from build123d import *

# Parameters (mm, degrees)
SKETCH2_W                     = 60
SKETCH2_H                     = 60
BOSS_EXTRUDE1_DEPTH           = 5
SKETCH5_W                     = 9
SKETCH5_H                     = 36
BOSS_EXTRUDE2_DEPTH           = 30
BOSS_EXTRUDE3_DEPTH           = 5
BOSS_EXTRUDE4_DEPTH           = 5
FILLET6_R                     = 7
SKETCH4_W                     = 2.25
SKETCH4_H                     = 5
M4_CLEARANCE_HOLE2_AT_2_COUNT = 2
M4_CLEARANCE_HOLE2_AT_2_PITCH = 70.710678119
M4_CLEARANCE_HOLE2_AT_3_COUNT = 2
M4_CLEARANCE_HOLE2_AT_3_PITCH = 50
M4_CLEARANCE_HOLE2_AT_4_COUNT = 2
M4_CLEARANCE_HOLE2_AT_4_PITCH = 50
SKETCH17_R                    = 4.5
CUT_EXTRUDE7_DEPTH            = 5
CUT_EXTRUDE8_DEPTH            = 3
RIB9_REACH                    = 57
SKETCH19_WALLS_W              = 3
SKETCH19_WALLS_H              = 168.00000011
FILLET7_R                     = 5
CUT_EXTRUDE10_DEPTH           = 1.5
FILLET8_R                     = 1
SKETCH23_R                    = 1.25
CUT_EXTRUDE12_DEPTH           = 76.663729878
CIRPATTERN2_COUNT             = 3
FILLET10_R                    = 2
SKETCH24_R                    = 8.875
CUT_EXTRUDE13_DEPTH           = 7
CUT_EXTRUDE14_DEPTH           = 7
FILLET11_R                    = 7
SKETCH27_W                    = 5
SKETCH27_H                    = 6.169574238
CUT_EXTRUDE17_DEPTH           = 7
CUT_EXTRUDE18_DEPTH           = 1.5
CUT_EXTRUDE19_DEPTH           = 1.5
FILLET13_R                    = 3


with BuildPart() as part:
    # Sketch2 → Boss-Extrude1 (new body)
    with BuildSketch(Plane(origin=(0, 0, 0), x_dir=(1, 0, 0), z_dir=(0, 1, 0))):
        Rectangle(SKETCH2_W, SKETCH2_H)
    extrude(amount=BOSS_EXTRUDE1_DEPTH)

    # Sketch5 → Boss-Extrude2 (add)
    with BuildSketch(Plane(origin=(0, 5, 0), x_dir=(1, 0, 0), z_dir=(0, 1, 0))):
        with Locations((-25.5, 0)):
            Rectangle(SKETCH5_W, SKETCH5_H)
    extrude(amount=BOSS_EXTRUDE2_DEPTH)

    # Sketch6 → Boss-Extrude3 (add)
    with BuildSketch(Plane.XY.offset(18)):
        Polygon((-21, 35), (30, 5), (-21, 5), align=None)
    extrude(amount=-BOSS_EXTRUDE3_DEPTH)

    # Sketch15 → Boss-Extrude4 (add)
    with BuildSketch(Plane(origin=(0, 0, -18), x_dir=(-1, 0, 0), z_dir=(0, 0, -1))):
        Polygon((21, 5), (21, 35), (-30, 5), align=None)
    extrude(amount=-BOSS_EXTRUDE4_DEPTH)

    # Fillet6
    fillet6_edges = [part.edges().sort_by_distance(p)[0] for p in [
        (0, 5, 18),
        (0, 5, -18),
    ]]
    fillet(fillet6_edges, radius=FILLET6_R)

    # Sketch4 → M4 Clearance Hole2 (revolve, cut)
    with BuildSketch(Plane(origin=(25, 5, -25), x_dir=(0, 0, 1), z_dir=(1, 0, 0))):
        with Locations((1.125, 2.5)):
            Rectangle(SKETCH4_W, SKETCH4_H)
    m4_clearance_hole2 = revolve(axis=Axis((25, 11.35, -25), (0, -1, 0)), mode=Mode.SUBTRACT)

    # M4 Clearance Hole2 at 2: M4 Clearance Hole2 ×2
    with Locations(*[Vector(-0.7071067811865476, 0, 0.7071067811865476) * (i * M4_CLEARANCE_HOLE2_AT_2_PITCH) for i in range(1, M4_CLEARANCE_HOLE2_AT_2_COUNT)]):
        add(m4_clearance_hole2, mode=Mode.SUBTRACT)

    # M4 Clearance Hole2 at 3: M4 Clearance Hole2 ×2
    with Locations(*[(-i * M4_CLEARANCE_HOLE2_AT_3_PITCH, 0, 0) for i in range(1, M4_CLEARANCE_HOLE2_AT_3_COUNT)]):
        add(m4_clearance_hole2, mode=Mode.SUBTRACT)

    # M4 Clearance Hole2 at 4: M4 Clearance Hole2 ×2
    with Locations(*[(0, 0, i * M4_CLEARANCE_HOLE2_AT_4_PITCH) for i in range(1, M4_CLEARANCE_HOLE2_AT_4_COUNT)]):
        add(m4_clearance_hole2, mode=Mode.SUBTRACT)

    # Sketch17 → Cut-Extrude7 (cut)
    with BuildSketch(Plane(origin=(0, 5, 0), x_dir=(1, 0, 0), z_dir=(0, 1, 0))):
        with Locations((25, -25)):
            Circle(SKETCH17_R)
        with Locations((-25, -25)):
            Circle(SKETCH17_R)
        with Locations((-25, 25)):
            Circle(SKETCH17_R)
        with Locations((25, 25)):
            Circle(SKETCH17_R)
    extrude(amount=CUT_EXTRUDE7_DEPTH, mode=Mode.SUBTRACT)

    # Sketch18 → Cut-Extrude8 (cut)
    with BuildSketch(Plane.XZ):
        with BuildLine():
            Line((-28, 21.989601355), (-28, -21.989601355))
            ThreePointArc((-28, -21.989601355), (-21.99479618, -21.99479618), (-21.989601355, -28))
            Line((-21.989601355, -28), (21.989601355, -28))
            ThreePointArc((21.989601355, -28), (21.99479618, -21.99479618), (28, -21.989601355))
            Line((28, -21.989601355), (28, 21.989601355))
            ThreePointArc((28, 21.989601355), (21.99479618, 21.99479618), (21.989601355, 28))
            Line((21.989601355, 28), (-21.989601355, 28))
            ThreePointArc((-21.989601355, 28), (-21.99479618, 21.99479618), (-28, 21.989601355))
        make_face()
    extrude(amount=-CUT_EXTRUDE8_DEPTH, mode=Mode.SUBTRACT)

    # Sketch19 walls → Rib9 (add, up to next)
    with BuildSketch(Plane.XZ, mode=Mode.PRIVATE) as rib9_sk1:
        with Locations((15.5, 0)):
            Rectangle(SKETCH19_WALLS_W, SKETCH19_WALLS_H)
    rib9_tool1 = extrude(rib9_sk1.sketch, amount=-RIB9_REACH, mode=Mode.PRIVATE) - part.part
    # Sketch19 walls → Rib9 (add, up to next)
    with BuildSketch(Plane.XZ, mode=Mode.PRIVATE) as rib9_sk2:
        with Locations((-15.5, 0)):
            Rectangle(SKETCH19_WALLS_W, SKETCH19_WALLS_H)
    rib9_tool2 = extrude(rib9_sk2.sketch, amount=-RIB9_REACH, mode=Mode.PRIVATE) - part.part
    add(rib9_tool1.solids().sort_by_distance((15.5, 0, 0))[0])
    add(rib9_tool2.solids().sort_by_distance((-15.5, 0, 0))[0])

    # Fillet7
    # the kernel refuses this fillet: 5 mm, written as the material it adds along each edge
    with BuildSketch(Plane(origin=(-21, 5, 13), x_dir=(1, 0, 0), z_dir=(0, 0, -1))) as fillet7_piece_1:
        with BuildLine():
            CenterArc((FILLET7_R, -FILLET7_R), FILLET7_R, 90, 90)
            Line((0, -FILLET7_R), (0, 0))
            Line((0, 0), (FILLET7_R, 0))
        make_face()
    extrude(amount=26)
    with BuildSketch(Plane(origin=(42.5, 5, 13), x_dir=(0, 0, -1), z_dir=(-1, 0, 0))) as fillet7_piece_2_section:
        with BuildLine():
            CenterArc((FILLET7_R, -FILLET7_R), FILLET7_R, 90, 90)
            Line((0, -FILLET7_R), (0, 0))
            Line((0, 0), (FILLET7_R, 0))
        make_face()
    fillet7_piece_2 = extrude(amount=63.5, mode=Mode.PRIVATE)
    fillet7_piece_2 = split(fillet7_piece_2, bisect_by=Plane(origin=(9.894433322, 16.826803928, 11.865257735), z_dir=(-0.5070201265633938, -0.8619342151577696, 0)), keep=Keep.TOP, mode=Mode.PRIVATE)
    add(fillet7_piece_2)
    with BuildSketch(Plane(origin=(42.5, 5, -13), x_dir=(0, 0, 1), z_dir=(-1, 0, 0))) as fillet7_piece_3_section:
        with BuildLine():
            CenterArc((FILLET7_R, FILLET7_R), FILLET7_R, 180, 90)
            Line((0, FILLET7_R), (0, 0))
            Line((0, 0), (FILLET7_R, 0))
        make_face()
    fillet7_piece_3 = extrude(amount=63.5, mode=Mode.PRIVATE)
    fillet7_piece_3 = split(fillet7_piece_3, bisect_by=Plane(origin=(9.894433322, 16.826803928, -11.865257735), z_dir=(-0.5070201265633937, -0.8619342151577696, 0)), keep=Keep.TOP, mode=Mode.PRIVATE)
    add(fillet7_piece_3)

    # Sketch21 → Cut-Extrude10 (cut)
    with BuildSketch(Plane.XY.offset(-13)):
        Polygon((-19, 31.503166715), (-19, 12), (14.155383415, 12), align=None)
    cut_extrude10 = extrude(amount=-CUT_EXTRUDE10_DEPTH, mode=Mode.SUBTRACT)

    # Fillet8
    fillet8_edges = [part.edges().sort_by_distance(p)[0] for p in [
        (-21, 22.5, 13),
        (-21, 22.5, -13),
        (-19.230244537, 6.183519916, 11.230244537),
        (-19.230244537, 6.183519916, -11.230244537),
    ]]
    fillet(fillet8_edges, radius=FILLET8_R)

    # Mirror3: Cut-Extrude10 across plane
    add(cut_extrude10.mirror(Plane.XY), mode=Mode.SUBTRACT)

    # Sketch23 → Cut-Extrude12 (cut, through all)
    with BuildSketch(Plane(origin=(-30, 0, 0), x_dir=(0, 0, -1), z_dir=(1, 0, 0))):
        with Locations(Location((0.544723392, 26.226216863, 0), (0, 0, 180))):
            Circle(SKETCH23_R)
    cut_extrude12 = extrude(amount=CUT_EXTRUDE12_DEPTH, mode=Mode.SUBTRACT)

    # CirPattern2: Cut-Extrude12 ×3 about axis
    cirpattern2_axis = Axis((0, 20, 0), (1, 0, 0))
    for i in range(1, CIRPATTERN2_COUNT):
        add(cut_extrude12.rotate(cirpattern2_axis, i * 360 / CIRPATTERN2_COUNT), mode=Mode.SUBTRACT)

    # Fillet10
    fillet10_edges = [part.edges().sort_by_distance(p)[0] for p in [
        (-30, 2.5, -30),
        (-30, 2.5, 30),
        (30, 2.5, 30),
        (30, 2.5, -30),
    ]]
    fillet(fillet10_edges, radius=FILLET10_R)

    # Sketch24 → Cut-Extrude13 (cut)
    with BuildSketch(Plane.ZY.offset(30)):
        with Locations((0, 20)):
            Circle(SKETCH24_R)
    extrude(amount=-CUT_EXTRUDE13_DEPTH, mode=Mode.SUBTRACT)

    # Sketch25 → Cut-Extrude14 (cut)
    with BuildSketch(Plane.ZY.offset(30)):
        Polygon((-1.486450158, 28.74963376), (-10.151392059, 38.373026676), (-17.792172557, 39.760209508), (-17.211267901, 32.016285915), (-8.546326, 22.392892999), align=None)
    extrude(amount=-CUT_EXTRUDE14_DEPTH, mode=Mode.SUBTRACT)

    # Fillet11
    fillet11_edges = [part.edges().sort_by_distance(p)[0] for p in [
        (-26.5, 28.74963376, -1.486450158),
        (-26.5, 22.392892999, -8.546326),
    ]]
    fillet(fillet11_edges, radius=FILLET11_R)

    # Sketch27 → Cut-Extrude17 (cut)
    with BuildSketch(Plane.ZY.offset(30)):
        with Locations((-15.5, 31.915212881)):
            Rectangle(SKETCH27_W, SKETCH27_H)
    extrude(amount=-CUT_EXTRUDE17_DEPTH, mode=Mode.SUBTRACT)

    # Sketch28 → Cut-Extrude18 (cut)
    with BuildSketch(Plane(origin=(0, 0, -18), x_dir=(-1, 0, 0), z_dir=(0, 0, -1))):
        Polygon((28, 14), (28, 26.830425762), (21, 26.830425762), (21, 32.679637303), (-10.755383415, 14), align=None)
    extrude(amount=-CUT_EXTRUDE18_DEPTH, mode=Mode.SUBTRACT)

    # Sketch29 → Cut-Extrude19 (cut)
    with BuildSketch(Plane.XY.offset(18)):
        Polygon((10.755383415, 14), (-21.544616585, 33), (-28, 33), (-28, 14), align=None)
    extrude(amount=-CUT_EXTRUDE19_DEPTH, mode=Mode.SUBTRACT)

    # Fillet13
    # the kernel refuses this fillet: 3 mm, written as the material it takes off along each edge
    with BuildSketch(Plane(origin=(-51.842425733, 35, -7.114305199), x_dir=(0, -0.6691623373486353, 0.7431162535391829), z_dir=(1, 0, 0))) as fillet13_piece_1:
        with BuildLine():
            CenterArc((7.536318289, -2.749260767), FILLET13_R, 66.408234173, 161.58931935)
            Line((5.528831277, -4.978609528), (5.328082575, -5.201544404))
            Line((5.328082575, -5.201544404), (-0.200748701, -0.222934876))
            Line((-0.200748701, -0.222934876), (-0.031345799, 0.298357907))
            ThreePointArc((-0.031345799, 0.298357907), (5.172701164, 0.845100622), (8.857035494, 0.274926077))
            Line((8.857035494, 0.274926077), (8.736970293, 0))
        make_face()
    extrude(amount=28.842425733, mode=Mode.SUBTRACT)


solid = part.part
Verification items for the finished model (mm, model axes). A direction names the side the tool comes from. Coordinates: 2 decimals unless noted, no trailing zeros. Write each loop counter-clockwise with the first axis right and the second up, starting at its lowest first coordinate (ties: lowest second). Pieces come first, ordered by that corner, then holes. Notation, with made-up numbers: M 8.5,-1.5 L 46.5,-1.5 A12 ccw 46.5,14.5 Z; hole C 64,-10.5 d6. An arc over 180 degrees is marked long. Use a Markdown table: item, result.
Q1. Go/stop test with flat-tipped pins: P1, Ø1, axis at x = -5.5, y = 11, coming from the +Z side; P2, Ø15.5, axis at x = 0.5, y = 17.5, coming from the -Z side; P3, Ø1, axis at x = -13, y = 19.5, coming from the -Z side; P4, Ø4, axis at x = -25, z = 25, coming from the +Y side. Record where each tip stops, or that it passes through.
Reply:
| item | result |
|---|---|
| P1 | stops at z = 18.16 |
| P2 | stops at z = -18.37 |
| P3 | stops at z = -16.5 |
| P4 | passes through |
Q2. Thickness scan on line 1 (X direction, y = 2.35, z = -25); line 2 (Z direction, x = 25, y = 1.2); line 3 (X direction, y = 3.5, z = -25). Record the ranges inside material, lowest first.
Reply:
| item | result |
|---|---|
| line 1 | x = -30 to -27.25, -22.75 to -20.75, -17 to -14, 14 to 17, 20.75 to 22.75, 27.25 to 30 |
| line 2 | z = -30 to -27.25, -22.75 to -20.75, 20.75 to 22.75, 27.25 to 30 |
| line 3 | x = -30 to -27.25, -22.75 to 22.75, 27.25 to 30 |
Q3. Set-up check for faces 4 (the face through (-26.55, 26.82, -12.53)), 5 (the face through (-8, 14, -17)), 6 (the face through (-2, 22, -13)): record each of +Z, -Z, +X, -X, +Y, -Y from which the full face is reachable in a straight line by a thin tool's end or side.
Reply:
| item | result |
|---|---|
| face 4 | -X, +Y |
| face 5 | -Z |
| face 6 | +X, +Y |
Q4. Sectioned sample at B-B, the plane x = 25. Record the boundary of the cut face in (y, z), plus the area to 3 significant figures.
Reply:
| item | result |
|---|---|
| outline | M 0,-30 L 5,-30 L 5,-27.25 L 0,-27.25 Z; M 0,-22.75 L 5,-22.75 L 5,-20.5 L 6.64,-20.5 A7 cw 7.94,-19.3 L 7.94,-12.56 A5 cw 5,-8 L 5,8 A5 cw 7.94,12.56 L 7.94,19.3 A7 cw 6.64,20.5 L 5,20.5 L 5,22.75 L 0,22.75 L 0,20.75 L 3,20.75 L 3,-20.75 L 0,-20.75 Z; M 0,27.25 L 5,27.25 L 5,30 L 0,30 Z |
| area | 183 mm² |
Q5. Sectioned sample at A-A, the plane y = 4. Record the boundary of the cut face in (x, z).
Reply:
| item | result |
|---|---|
| outline | M -30,-28 A2 ccw -28,-30 L 28,-30 A2 ccw 30,-28 L 30,28 A2 ccw 28,30 L -28,30 A2 ccw -30,28 Z; hole C -25,-25 d4.5; hole C -25,25 d4.5; hole C 25,-25 d4.5; hole C 25,25 d4.5 |
Q6. Draft check along X on faces 1 (the face through (5, 6, 11)), 2 (the face through (-23, 23, -5)), 3 (the face through (-3, 12, -14)). Enter one of: +X half, -X half, draft (parallel to the pull), parting line (faces both ways), or undercut.
Reply:
| item | result |
|---|---|
| face 1 | draft |
| face 2 | -X half |
| face 3 | undercut |
